The figure shows three views and two pictorial views of one solid part (mm, origin at its lowest corner). Answer the questions. Give positions to 0.01 mm unless a question says otherwise; leave off trailing zeros. Order: outer loops, then holes, each group sorted by start corner. A loop starts at its lowest first (then second) coordinate and runs counter-clockwise, first axis right, second up. Notation, with made-up numbers: (-4, -12) - (52, -12) arc R29 ccw to (52, 25) - close; hole circle Ø4 at (-11.5, -32.75). An arc over 180 degrees is marked (long way). Write item = value, one per line.
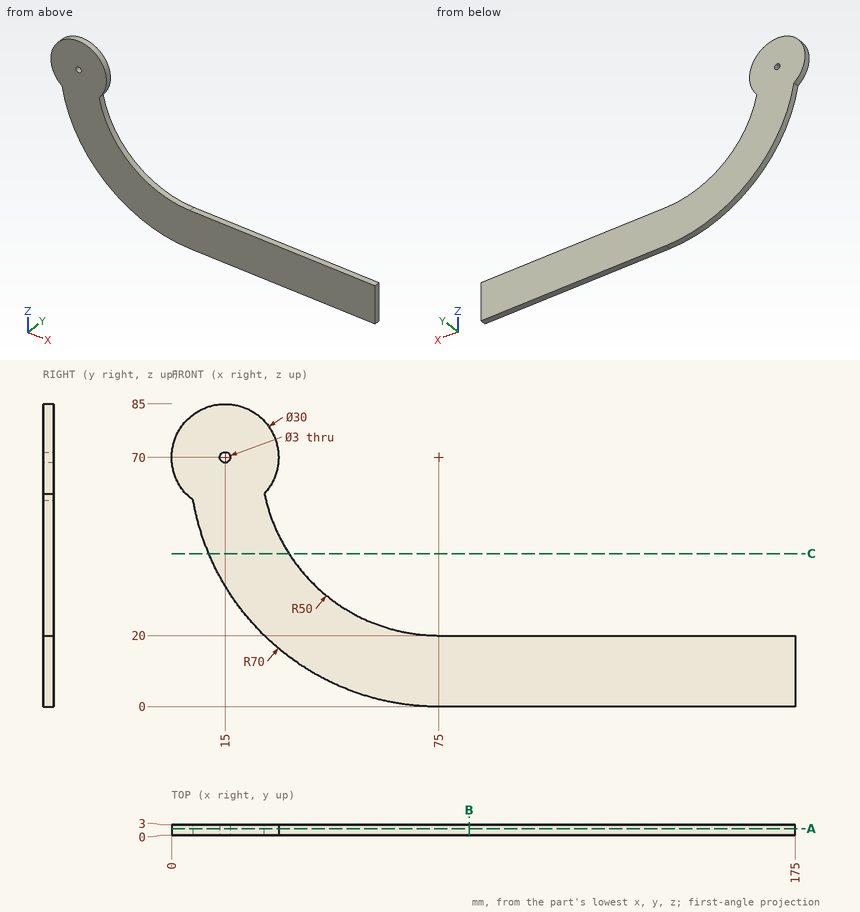
1. Flat-ended cylindrical pins translate along their axes: pin 1 (1.5 mm diameter, centred on x = 64, y = 0.5, fed in from -Z); pin 2 (1 mm diameter, centred on y = 1.5, z = 35, fed in from +X); pin 3 (5 mm diameter, centred on x = 15, z = 70, fed in from +Y). Find the tip coordinate at first contact, or state that the pin passes through.
Recorded:
pin_1 = 0.75
pin_2 = 39.79
pin_3 = 3
2. Section B-B (x = 83.5) is taken. Determine the outline of the cut face in (y, z).
Recorded:
outline = (0, 0) - (3, 0) - (3, 20) - (0, 20) - close
3. Section A-A (y = 1.9) is taken. Determine the outline of the cut face in (x, z), and give its area (3 significant figures).
Recorded:
outline = (6.04, 57.97) arc R70 ccw to (75, 0) - (175, 0) - (175, 20) - (75, 20) arc R50 cw to (26.04, 59.85) arc R15 ccw (long way) to start; hole circle Ø3 at (15, 70)
area = 4,310 mm^2
4. Straight lines are drawn through the part: L1, parallel to X at y = 0.8, z = 70; L2, parallel to Z at x = 115, y = 2.35; L3, parallel to Z at x = 15, y = 2. For each, find the intervals that lie inside material, in ascending order. Write a range as [from, to].
Recorded:
L1 = [0, 13.5], [16.5, 30]
L2 = [0, 20]
L3 = [33.94, 68.5], [71.5, 85]
5. Section C-C (z = 43) is taken. Determine the outline of the cut face in (x, y).
Recorded:
outline = (10.42, 0) - (32.92, 0) - (32.92, 3) - (10.42, 3) - close
